Work out the finished part from the listing and answer in its coordinate system (mm). A direction names the side the tool comes from. Coordinates: 2 decimals unless noted, no trailing zeros. Order: outer loops, then holes, each group sorted by start corner. A loop starts at its lowest first (then second) coordinate and runs counter-clockwise, first axis right, second up. Notation, with made-up numbers: M -9.5,-2.75 L 37.5,-2.75 A11 cw 37.5,11.25 Z; hole C -33.75,10.5 d4. An arc over 180 degrees is marked long. Use a Markdown table: item, result. Add a question column.
from build123d import *

# Parameters (mm, degrees)
F1_DEPTH = 54
F2_DEPTH = 54
F4_D     = 3.2
F4_DEPTH = 14.25
F4_TIP   = 0.9613769904


# Not quite as in the source:
# - ends of sketch curves that miss each other by under 0.0002 mm in the source are joined


with BuildPart() as f1:
    # F0 (on Front) → F1 (new body)
    with BuildSketch(Plane.XZ):
        with BuildLine():
            Line((-15.9999975914, -11.0858444687), (-13.9999981419, -11.0858444687))
            Line((-13.9999981419, -11.0858444687), (-14.9999975913, -10.0858455697))
            Line((-14.9999975913, -10.0858455697), (-14.9999975913, 8.4141544303))
            Line((-14.9999975913, 8.4141544303), (-13.9999975913, 9.4141544303))
            Line((-13.9999975913, 9.4141544303), (14.0000024087, 9.4141544303))
            Line((14.0000024087, 9.4141544303), (15.0000024087, 8.4141544303))
            Line((15.0000024087, 8.4141544303), (15.0000024087, -10.0858455697))
            Line((15.0000024087, -10.0858455697), (14.0000024087, -11.0858455697))
            Line((14.0000024087, -11.0858455697), (16.0000024087, -11.0858444685))
            Line((16.0000024087, -11.0858444685), (16.7000024086, -10.3858444685))
            Line((16.7000024086, -10.3858444685), (16.7000024087, 3.914155003))
            Line((16.7000024087, 3.914155003), (17.0000024087, 4.2141550029))
            Line((17.0000024087, 4.2141550029), (17.0000024088, 13.3141544304))
            Line((17.0000024088, 13.3141544304), (16.4000024089, 13.9141544303))
            Line((16.4000024089, 13.9141544303), (7.9944513482, 13.9141544304))
            ThreePointArc((7.9944513482, 13.9141544304), (7.3786811713, 13.5433235007), (6.671572232, 13.4141513784))
            Line((6.671572232, 13.4141513784), (4.8284325856, 13.4141513784))
            ThreePointArc((4.8284325856, 13.4141513784), (4.1213236463, 13.5433235007), (3.5055534694, 13.9141544304))
            Line((3.5055534694, 13.9141544304), (-3.5055486519, 13.9141544303))
            ThreePointArc((-3.5055486519, 13.9141544303), (-4.1213188288, 13.5433235006), (-4.828427768, 13.4141513784))
            Line((-4.828427768, 13.4141513784), (-6.6715674144, 13.4141513784))
            ThreePointArc((-6.6715674144, 13.4141513784), (-7.3788732943, 13.5428024468), (-7.9944465306, 13.9141544304))
            Line((-7.9944465306, 13.9141544304), (-16.3999975914, 13.9141544303))
            Line((-16.3999975914, 13.9141544303), (-16.9999975913, 13.3141544304))
            Line((-16.9999975913, 13.3141544304), (-16.9999975913, 4.2141550029))
            Line((-16.9999975913, 4.2141550029), (-16.6999975912, 3.9141550028))
            Line((-16.6999975912, 3.9141550028), (-16.6999975914, -10.3858444687))
            Line((-16.6999975914, -10.3858444687), (-15.9999975914, -11.0858444687))
        make_face()
    extrude(amount=-F1_DEPTH)

    # F0 (on Front) → F2 (join)
    with BuildSketch(Plane.XZ):
        with BuildLine():
            Line((-13.9999975913, -11.0858455697), (-6.9999968681, -11.0858455697))
            Line((-6.9999968681, -11.0858455697), (-5.5999972297, -9.6858459313))
            Line((-5.5999972297, -9.6858459313), (-5.5999972297, -6.2358522996))
            Line((-5.5999972297, -6.2358522996), (-6.3686160385, -5.4672334908))
            ThreePointArc((-6.3686160385, -5.4672334908), (-6.7178259107, -4.9036746123), (-7.2813847892, -4.5544647401))
            Line((-7.2813847892, -4.5544647401), (-7.4999972297, -4.3358522996))
            Line((-7.4999972297, -4.3358522996), (-7.4999972297, -2.435839563))
            Line((-7.4999972297, -2.435839563), (-7.2813847892, -2.2172271225))
            ThreePointArc((-7.2813847892, -2.2172271225), (-6.7178259107, -1.8680172504), (-6.3686160385, -1.3044583718))
            Line((-6.3686160385, -1.3044583718), (-6.150003598, -1.0858459313))
            Line((-6.150003598, -1.0858459313), (6.1500091386, -1.0858459313))
            Line((6.1500091386, -1.0858459313), (6.3686215791, -1.3044583718))
            ThreePointArc((6.3686215791, -1.3044583718), (6.7178314512, -1.8680172504), (7.2813903298, -2.2172271225))
            Line((7.2813903298, -2.2172271225), (7.5000027703, -2.435839563))
            Line((7.5000027703, -2.435839563), (7.5000027704, -4.3358522996))
            Line((7.5000027704, -4.3358522996), (7.2813903299, -4.5544647401))
            ThreePointArc((7.2813903299, -4.5544647401), (6.7178314513, -4.9036746123), (6.3686215792, -5.4672334908))
            Line((6.3686215792, -5.4672334908), (5.6000027704, -6.2358522996))
            Line((5.6000027704, -6.2358522996), (5.6000027703, -9.6858459313))
            Line((5.6000027703, -9.6858459313), (7.0000024087, -11.0858455697))
            Line((7.0000024087, -11.0858455697), (14.0000024087, -11.0858455697))
            Line((14.0000024087, -11.0858455697), (15.0000024087, -10.0858455697))
            Line((15.0000024087, -10.0858455697), (15.0000024087, 8.4141544303))
            Line((15.0000024087, 8.4141544303), (14.0000024087, 9.4141544303))
            Line((14.0000024087, 9.4141544303), (-13.9999975913, 9.4141544303))
            Line((-13.9999975913, 9.4141544303), (-14.9999975913, 8.4141544303))
            Line((-14.9999975913, 8.4141544303), (-14.9999975913, -10.0858455697))
            Line((-14.9999975913, -10.0858455697), (-13.9999975913, -11.0858455697))
        make_face()
    extrude(amount=-F2_DEPTH)

    # F4
    with Locations(Plane.XY.offset(13.9141544304)):
        with Locations((13.0000000001, 14), (-12.9999999999, 14), (-12.9999999999, 40), (13.0000000001, 40)):
            Hole(F4_D / 2, depth=F4_DEPTH)
            with Locations((0, 0, -(F4_DEPTH + F4_TIP / 2))):  # 118° drill point
                Cone(0, F4_D / 2, F4_TIP, mode=Mode.SUBTRACT)


solid = f1.part
(1) A cutting plane is placed at C-C on z = 12. Write down the section's boundary in (x, y), plus the area to 3 significant figures.
(2) Which of the six approach directions +Z, -Z, +X, -X, +Y, -Y give full straight-line access (tool end or side, diameter ignored) to faces 1 (the cylindrical face through (13.208, 15.586, 6.689)), 2 (the cylindrical face through (-7.37, 26.62, 13.54)), 3 (the flat face through (-7.5, 27, -3)), 4 (the flat face through (5.6, 27, -8))?
(3) Given P1, Ø4, axis at y = 30, z = -7.5, coming from the +X side; P2, Ø1.5, axis at x = 1.5, y = 32, coming from the -Z side; P3, Ø0.9, axis at x = 5.5, y = 15.5, coming from the +Z side, each flat-ended and moving along its own axis, determine where each tip first touches the part or whether it passes through.
(4) A cutting plane is placed at A-A on z = 0.5. Write down the section's boundary in (x, y), plus the area to 3 significant figures.
(5) The mould has two halves that part along Z. Classify faces 5 (the flat face through (0, 27, 13.914)), 6 (the flat face through (-17, 27, 9)), 7 (the flat face through (7.5, 27, -3)): pulls with the +Z half, pulls with the -Z half, needs draft (parallel to the pull), parting line crosses it, or undercut.
(6) Straight lines are drawn through the part: line 1 (X direction, y = 14, z = 11); line 2 (Y direction, x = 13, z = 7); line 3 (X direction, y = 8.5, z = -7.25). For each, find the intervals that lie inside material, in ascending order.
(7) A cutting plane is placed at B-B on x = -1.5. Write down the section's boundary in (y, z).
From the geometry:
| question | item | result |
|---|---|---|
| 1 | outline | M -17,0 L 17,0 L 17,54 L -17,54 Z; hole C -13,14 d3.2; hole C -13,40 d3.2; hole C 13,14 d3.2; hole C 13,40 d3.2 |
| 1 | area | 1,800 mm2 |
| 2 | face 1 | +Z |
| 2 | face 2 | +Z, +Y, -Y |
| 2 | face 3 | +Y, -Y |
| 2 | face 4 | -Z, +Y, -Y |
| 3 | P1 | stops at x = 16.7 |
| 3 | P2 | stops at z = -1.09 |
| 3 | P3 | stops at z = 13.41 |
| 4 | outline | M -16.7,0 L 16.7,0 L 16.7,54 L -16.7,54 Z; hole C -13,14 d3.2; hole C -13,40 d3.2; hole C 13,14 d3.2; hole C 13,40 d3.2 |
| 4 | area | 1,770 mm2 |
| 5 | face 5 | pulls with the +Z half |
| 5 | face 6 | needs draft |
| 5 | face 7 | undercut |
| 6 | line 1 | x = -17 to -14.6, -11.4 to 11.4, 14.6 to 17 |
| 6 | line 2 | y = 0 to 12.4, 15.6 to 38.4, 41.6 to 54 |
| 6 | line 3 | x = -16.7 to -5.6, 5.6 to 16.7 |
| 7 | outline | M 0,-1.09 L 54,-1.09 L 54,13.91 L 0,13.91 Z |
